from build123d import *

# Parameters (mm, degrees)
SKETCH_6_R               = 5
SKETCH_8_W               = 10
SKETCH_8_H               = 10
EXTRUDE_1_DEPTH          = 7.5
SKETCH_9_R               = 5
EXTRUDE_2_DEPTH          = 5
SKETCH_11_R              = 60
EXTRUDE_3_DEPTH          = 45
PATTERN_CIRCULAR_1_COUNT = 6


with BuildPart() as part:
    # 掃出1: sweep along a path in 草圖7
    with BuildLine(Plane.XY) as sweep_1_path:
        Line((0, 0), (0, 130))
    # 草圖6 → 掃出1 (sweep)
    with BuildSketch(Plane(origin=(0, 0, 0), x_dir=(1, 0, 0), z_dir=(0, 1, 0))):
        Circle(SKETCH_6_R)
    sweep_1 = sweep(path=sweep_1_path.line)

    # 草圖8 → 填料-伸長1 (add, symmetric)
    with BuildSketch(Plane.XZ):
        Rectangle(SKETCH_8_W, SKETCH_8_H)
    extrude_1 = extrude(amount=EXTRUDE_1_DEPTH, both=True)

    # 草圖9 → 填料-伸長2 (add, symmetric)
    with BuildSketch(Plane.XY.offset(5)):
        with Locations((0, -0.5)):
            Circle(SKETCH_9_R)
    extrude_2 = extrude(amount=EXTRUDE_2_DEPTH, both=True)

    # 草圖11 → 填料-伸長3 (add, symmetric)
    with BuildSketch(Plane.XY):
        with Locations((0, 130)):
            Circle(SKETCH_11_R)
    extrude(amount=EXTRUDE_3_DEPTH, both=True)

    # 環狀複製排列1: 掃出1, 填料-伸長1, 填料-伸長2 ×6 about axis
    pattern_circular_1_axis = Axis((0, 130, 0), (0, 0, 1))
    add([sweep_1.rotate(pattern_circular_1_axis, i * 360 / PATTERN_CIRCULAR_1_COUNT) for i in range(1, PATTERN_CIRCULAR_1_COUNT)])
    add([extrude_1.rotate(pattern_circular_1_axis, i * 360 / PATTERN_CIRCULAR_1_COUNT) for i in range(1, PATTERN_CIRCULAR_1_COUNT)])
    add([extrude_2.rotate(pattern_circular_1_axis, i * 360 / PATTERN_CIRCULAR_1_COUNT) for i in range(1, PATTERN_CIRCULAR_1_COUNT)])


solid = part.part
Geometry check sheet. Reference: the model listing, model coordinates, mm. A direction names the side the tool comes from. Give positions to 0.01 mm unless a question says otherwise; leave off trailing zeros. Order: outer loops, then holes, each group sorted by start corner. A loop starts at its lowest first (then second) coordinate and runs counter-clockwise, first axis right, second up.
1) Cross-section at B-B (z = -31). Record the boundary of the cut face in (x, y), then the cut area to 3 significant figures.
Results are:
outline: circle Ø120 at (0, 130)
area: 11,300 mm2
2) Cross-section at A-A (y = 130). Record the boundary of the cut face in (x, z), then the cut area to 3 significant figures.
Results are:
outline: (-60, -45) - (60, -45) - (60, 45) - (-60, 45) - close
area: 10,800 mm2
3) Material ranges on probe 1 along Y at (x, z) = (1, -25.5); probe 2 along Y at (x, z) = (36, 17); probe 3 along X at (y, z) = (153, -8), recorded low to high.
Results are:
probe 1: y = 70.01 to 189.99
probe 2: y = 82 to 178
probe 3: x = -55.42 to 55.42
4) Gauge pin test, flat ends, axial feed: pin 1 (4 mm diameter, centred on x = 14, z = 15.5, fed in from -Y); pin 2 (11 mm diameter, centred on x = -115.5, y = 63.5, fed in from +Z); pin 3 (1.5 mm diameter, centred on y = 226.5, z = 1, fed in from +X). Record the tip position at first contact, or that the pin passes through.
Results are:
pin 1: stops at y = 71.21
pin 2: stops at z = 10
pin 3: stops at x = 4.99
5) Draft check along Y on faces 6 (the cylindrical face through (-80.9, 171.2, -1.5)), 7 (the flat face through (113, 65, -5)), 8 (the flat face through (-119.043, 198.811, 0.07)). Enter one of: released by +Y, released by -Y, zero draft, split by the parting line, or undercut.
Results are:
face 6: undercut
face 7: zero draft
face 8: released by +Y
6) Cross-section at D-D (y = 77). Give the number of separate pieces and of enclosed holes in the cut face, then the cut area to 3 significant figures.
Results are:
separate pieces: 3
enclosed holes: 0
area: 5,380 mm2
7) Cross-section at C-C (x = 41). Record the boundary of the cut face in (y, z), then the cut area to 3 significant figures.
Results are:
outline: (86.19, -45) - (173.81, -45) - (173.81, 45) - (86.19, 45) - close
area: 7,890 mm2
8) Tool access check on faces 1 (the flat face through (0, 260, 10)), 2 (the cylindrical face through (-1.08, -5.38, 7.54)), 3 (the flat face through (119.113, 198.689, 0.07)), 4 (the flat face through (0, 0, -5)), 5 (the flat face through (-110.17, 60.62, -0.07)). Record the directions out of +Z, -Z, +X, -X, +Y, -Y that give a thin tool (end or side, any length) a straight path to the whole face; none if there is none.
Results are:
face 1: +Z, +X, -X, +Y
face 2: +Z
face 3: +Z, -Z, +X, +Y
face 4: -Z, +X, -X, -Y
face 5: +Z, -Z, -Y
